Geometry: final body of the model. Coordinates: model frame, mm. A direction names the side the tool comes from. Give positions to 0.01 mm unless a question says otherwise; leave off trailing zeros. Loops run counter-clockwise (first coordinate to the right, second up) from the corner with the lowest first, then second, coordinate; pieces in that order, holes last. Notation, with made-up numbers: (65, 73.5) -> (98, 73.5) arc R18 ccw to (98, 85.5) -> close; hole circle Ø8 at (74, -38). An arc over 180 degrees is marked (long way). Answer in a Markdown table with one row per item. Add a question column.
1) Line query: line 1 (Y direction, x = 0, z = -42); line 2 (Z direction, x = 1.5, y = 7.5) (1 decimal); line 3 (Y direction, x = 34.5, z = -10.5). Output: solid intervals per line, ascending. Write a range as from..to.
2) Section query B-B (z = 0). Return the cut outline in (x, y).
3) First-contact query: P1, Ø1, axis at y = 8, z = -17.5, coming from the +X side; P2, Ø6.5, axis at x = 0, z = 0, coming from the -Y side; P3, Ø10, axis at x = -3, z = -3.5, coming from the -Y side; P4, Ø2, axis at x = -2, y = 5, coming from the +Z side. Flat tips, straight axial feed; report the tip coordinate or a pass-through.
4) Section query D-D (z = -32.5). Return the cut outline in (x, y).
5) Section query A-A (x = 0). Return the cut outline in (y, z), plus the area to 3 significant figures.
6) Draft query along Y for faces 1 (the cylindrical face through (-0.751, 7.385, -42.425)), 2 (the flat face through (4, 5, -4)), 3 (the flat face through (1, 10, -9)), 4 (the cylindrical face through (5.37, 7.54, 1.19)). Return one class per face: +Y half, -Y half, draft (parallel to the pull), parting line (faces both ways), or undercut.
7) Access query for faces 5 (the flat face through (8, 8, -8)), 6 (the cylindrical face through (-0.751, 2.615, 42.425)), 7 (the flat face through (30.2, 0, -26.5)). Directions: +Z, -Z, +X, -X, +Y, -Y. A direction counts if a zero-diameter tool reaches every point of the face in a straight line with its end or side. Return the directions, or none.
Autodesk Inventor part; units mm, degrees
ref_plane "Work Plane1" through (0, 0, 45) normal (0, 0, 1) x (1, 0, 0)
ref_plane "Work Plane2" through (0, 0, -45) normal (0, 0, 1) x (1, 0, 0)
ref_plane "YZ Plane" through (0, 0, 0) normal (1, 0, 0) x (0, 1, 0)
sketch "Sketch1" plane through (0, 0, 0) normal (0, 1, 0) x (-1, 0, 0)
  circle A0 centre (0, 0) radius 45
  dimension "d0" = 90
extrude "Extrusion1" add sketch "Sketch1" along normal blind 10
sketch "Sketch2" plane through (0, 0, 0) normal (0, -1, 0) x (1, 0, 0)
  circle A0 centre (0, 0) radius 45
  circle A1 centre (0, 0) radius 40
  dimension "d3" = 80
extrude "Extrusion2" cut sketch "Sketch2" against normal blind 5 contours A1
sketch "Sketch3" plane through (0, 5, 0) normal (0, -1, 0) x (1, 0, 0)
  circle A0 centre (0, 0) radius 40
  circle A1 centre (0, 0) radius 10
  dimension "d6" = 20
extrude "Extrusion3" cut sketch "Sketch3" against normal blind 3
sketch "Sketch4" plane through (0, 5, 0) normal (0, -1, 0) x (1, 0, 0)
  circle A0 centre (0, 0) radius 10
hole "Hole1" at (0, 5, 0) direction (0, 1, 0) diameter 11 end through all
ref_plane "Work Plane1" through (0, 0, 45) normal (0, 0, 1) x (1, 0, 0)
sketch "Sketch5" plane through (0, 0, 45) normal (0, 0, 1) x (1, 0, 0)
  point P0 (0, 0)
  point P1 (0, 5)
  dimension "d17" = 5
ref_plane "Work Plane2" through (0, 0, -45) normal (0, 0, 1) x (1, 0, 0)
sketch "Sketch6" plane through (0, 0, -45) normal (0, 0, 1) x (1, 0, 0)
  point P0 (0, 0)
  point P1 (0, 5)
  dimension "d19" = 5
hole "Hole2" at (0, 5, 45) direction (0, 0, -1) diameter 5 depth 8 tip angle 118
hole "Hole3" at (0, 5, -45) direction (0, 0, 1) diameter 5 depth 8 tip angle 118
properties part number "rotor" material "PMMA Plastic"
Evaluation:
| question | item | result |
|---|---|---|
| 1 | line 1 | 0..2.5, 7.5..10 |
| 1 | line 2 | -45..-40, -9.9..-5.3, 5.3..9.9, 40..45 |
| 1 | line 3 | 8..10 |
| 2 | outline | (-45, 0) -> (-40, 0) -> (-40, 8) -> (-10, 8) -> (-10, 5) -> (-5.5, 5) -> (-5.5, 10) -> (-45, 10) -> close; (5.5, 5) -> (10, 5) -> (10, 8) -> (40, 8) -> (40, 0) -> (45, 0) -> (45, 10) -> (5.5, 10) -> close |
| 3 | P1 | x = 41.67 |
| 3 | P2 | through |
| 3 | P3 | y = 5 |
| 3 | P4 | z = 44.94 |
| 4 | outline | (-31.12, 0) -> (-23.32, 0) -> (-23.32, 8) -> (23.32, 8) -> (23.32, 0) -> (31.12, 0) -> (31.12, 10) -> (-31.12, 10) -> close |
| 5 | outline | (0, -45) -> (2.5, -45) -> (2.5, -40) -> (0, -40) -> close; (0, 40) -> (2.5, 40) -> (2.5, 45) -> (0, 45) -> close; (5, -10) -> (8, -10) -> (8, -40) -> (7.5, -40) -> (7.5, -45) -> (10, -45) -> (10, -5.5) -> (5, -5.5) -> close; (5, 5.5) -> (10, 5.5) -> (10, 45) -> (7.5, 45) -> (7.5, 40) -> (8, 40) -> (8, 10) -> (5, 10) -> close |
| 5 | area | 215 mm² |
| 6 | face 1 | undercut |
| 6 | face 2 | -Y half |
| 6 | face 3 | +Y half |
| 6 | face 4 | draft |
| 7 | face 5 | -Y |
| 7 | face 6 | +Z |
| 7 | face 7 | +Z, -Z, +X, -X, -Y |
